from build123d import *

# Parameters (mm, degrees)
F0_W         = 190
F0_H         = 190
F0_W_2       = 11
F0_H_2       = 115.8
F0_R         = 2.1
F0_W_3       = 0.5
F0_H_3       = 0.5
F1_DEPTH     = 10
F0_W_4       = 5.2
F0_H_4       = 110
F2_DEPTH     = 5
F3_R         = 2.59999
F4_R         = 5.49999
F6_DEPTH     = 25
F8_R         = 6
F7_W         = 0.5
F7_H         = 29.5
F9_DEPTH     = 0.5
F7_W_2       = 15.563522011
F7_H_2       = 0.5
F10_DEPTH    = 0.5
F11_T2_ANGLE = 359.64
F11_T4_ANGLE = 293.7301704478
F11_T6_ANGLE = 293.7301704478


# Not quite as in the source:
# - a fillet or chamfer that OpenCascade refuses, or shapes differently, is made with other operations: its cross-section is extruded or revolved along the edge and cut away or added
# - a fillet or chamfer is up to 0.001 mm smaller than in the source, because OpenCascade refuses the exact size
# - ends of sketch curves that miss each other by under 0.0002 mm in the source are joined


with BuildPart() as f1:
    # F0 (on Top) → F1 (new body)
    with BuildSketch(Plane.XY):
        Rectangle(F0_W, F0_H)
        with BuildLine():
            ThreePointArc((50, -55), (47.0710678119, -62.0710678119), (40, -65))
            Line((40, -65), (0.25, -65))
            Line((0.25, -65), (0.25, -65.5))
            Line((0.25, -65.5), (-0.25, -65.5))
            Line((-0.25, -65.5), (-0.25, -65))
            Line((-0.25, -65), (-40, -65))
            ThreePointArc((-40, -65), (-47.0710678119, -62.0710678119), (-50, -55))
            Line((-50, -55), (-50, 55))
            ThreePointArc((-50, 55), (-47.0710678119, 62.0710678119), (-40, 65))
            Line((-40, 65), (-21, 65))
            ThreePointArc((-21, 65), (-13.9289321881, 62.0710678119), (-11, 55))
            Line((-11, 55), (-11, -9))
            ThreePointArc((-11, -9), (-7.8660663613, -16.6892782496), (-0.25, -19.997158724))
            Line((-0.25, -19.997158724), (-0.25, -19.5))
            Line((-0.25, -19.5), (0.25, -19.5))
            Line((0.25, -19.5), (0.25, -19.997158724))
            ThreePointArc((0.25, -19.997158724), (7.8660663613, -16.6892782496), (11, -9))
            Line((11, -9), (11, 55))
            ThreePointArc((11, 55), (13.9289321881, 62.0710678119), (21, 65))
            Line((21, 65), (40, 65))
            ThreePointArc((40, 65), (47.0710678119, 62.0710678119), (50, 55))
            Line((50, 55), (50, -55))
        make_face(mode=Mode.SUBTRACT)
        with Locations((-73.936477989, 0)):
            Rectangle(F0_W_2, F0_H_2, mode=Mode.SUBTRACT)
        Circle(F0_R, mode=Mode.SUBTRACT)
        with Locations((73.936477989, 0)):
            Rectangle(F0_W_2, F0_H_2, mode=Mode.SUBTRACT)
        with BuildLine():
            ThreePointArc((0, -20), (0.1250080726, -19.9992896581), (0.25, -19.997158724))
            Line((0.25, -19.997158724), (0.25, -19.5))
            Line((0.25, -19.5), (-0.25, -19.5))
            Line((-0.25, -19.5), (-0.25, -19.997158724))
            ThreePointArc((-0.25, -19.997158724), (-0.1250080726, -19.9992896581), (0, -20))
        make_face()
        with Locations((0, -65.25)):
            Rectangle(F0_W_3, F0_H_3)
    extrude(amount=F1_DEPTH)

    # F0 (on Top) → F2 (join)
    with BuildSketch(Plane.XY):
        with Locations((-73.936477989, 0)):
            Rectangle(F0_W_2, F0_H_2)
        with Locations((-73.936477989, 0)):
            Rectangle(F0_W_4, F0_H_4, mode=Mode.SUBTRACT)
        with Locations((73.936477989, 0)):
            Rectangle(F0_W_2, F0_H_2)
        with Locations((73.936477989, 0)):
            Rectangle(F0_W_4, F0_H_4, mode=Mode.SUBTRACT)
    extrude(amount=F2_DEPTH)

    # F3 (radius 2.6 in the source; OpenCascade refuses exactly that, so slightly less here)
    f3_edges = [f1.edges().sort_by_distance(p)[0] for p in [
        (-76.536478, 55, 2.5),
        (-71.336478, 55, 2.5),
        (-76.536478, -55, 2.5),
        (-71.336478, -55, 2.5),
        (76.536478, -55, 2.5),
        (71.336478, -55, 2.5),
        (71.336478, 55, 2.5),
        (76.536478, 55, 2.5),
    ]]
    fillet(f3_edges, radius=F3_R)

    # F4 (radius 5.5 in the source; OpenCascade refuses exactly that, so slightly less here)
    f4_edges = [f1.edges().sort_by_distance(p)[0] for p in [
        (-79.436478, 57.9, 7.5),
        (-68.436478, 57.9, 7.5),
        (79.436478, 57.9, 7.5),
        (68.436478, 57.9, 7.5),
        (68.436478, -57.9, 7.5),
        (79.436478, -57.9, 7.5),
        (-79.436478, -57.9, 7.5),
        (-68.436478, -57.9, 7.5),
    ]]
    fillet(f4_edges, radius=F4_R)

    # F5 (on face) → F6 (cut)
    with BuildSketch(Plane.XY.offset(5)):
        with BuildLine():
            Line((-73.686477989, -55.5), (-73.686477989, -54.9879537784))
            ThreePointArc((-73.686477989, -54.9879537784), (-73.8113279558, -54.9969866984), (-73.936467989, -55))
            ThreePointArc((-73.936467989, -55), (-74.0616280221, -54.9969866984), (-74.186477989, -54.9879537784))
            Line((-74.186477989, -54.9879537784), (-74.186477989, -55.5))
            Line((-74.186477989, -55.5), (-73.686477989, -55.5))
        make_face()
        with BuildLine():
            ThreePointArc((-73.936467989, 55), (-73.8113279558, 54.9969866984), (-73.686477989, 54.9879537784))
            Line((-73.686477989, 54.9879537784), (-73.686477989, 55.5))
            Line((-73.686477989, 55.5), (-74.186477989, 55.5))
            Line((-74.186477989, 55.5), (-74.186477989, 54.9879537784))
            ThreePointArc((-74.186477989, 54.9879537784), (-74.0616280221, 54.9969866984), (-73.936467989, 55))
        make_face()
    extrude(amount=-F6_DEPTH, mode=Mode.SUBTRACT)

    # F8
    f8_edges = [f1.edges().sort_by_distance(p)[0] for p in [
        (-95, -95, 5),
        (95, -95, 5),
        (95, 95, 5),
        (-95, 95, 5),
    ]]
    fillet(f8_edges, radius=F8_R)

    # F7 (on face) → F9 (cut)
    with BuildSketch(Plane.XY.offset(10)):
        with BuildLine():
            Line((-0.25, 95), (-0.25, 2.0850659462))
            ThreePointArc((-0.25, 2.0850659462), (0, 2.1), (0.25, 2.0850659462))
            Line((0.25, 2.0850659462), (0.25, 95))
            Line((0.25, 95), (-0.25, 95))
        make_face()
        with BuildLine():
            Line((-0.25, -2.0850659462), (-0.25, -19.6))
            Line((-0.25, -19.6), (0.25, -19.6))
            Line((0.25, -19.6), (0.25, -2.0850659462))
            ThreePointArc((0.25, -2.0850659462), (0, -2.1), (-0.25, -2.0850659462))
        make_face()
        with Locations((0, -80.25)):
            Rectangle(F7_W, F7_H)
        with BuildLine():
            Line((-0.25, -0.25), (-0.25, -2.0850659462))
            ThreePointArc((-0.25, -2.0850659462), (0, -2.1), (0.25, -2.0850659462))
            Line((0.25, -2.0850659462), (0.25, -0.25))
            Line((0.25, -0.25), (-0.25, -0.25))
        make_face()
        with BuildLine():
            Line((-0.25, 2.0850659462), (-0.25, 0.25))
            Line((-0.25, 0.25), (0.25, 0.25))
            Line((0.25, 0.25), (0.25, 2.0850659462))
            ThreePointArc((0.25, 2.0850659462), (0, 2.1), (-0.25, 2.0850659462))
        make_face()
    extrude(amount=-F9_DEPTH, mode=Mode.SUBTRACT)

    # F7 (on face) → F10 (cut)
    with BuildSketch(Plane.XY.offset(10)):
        with Locations((87.2182389945, 0)):
            Rectangle(F7_W_2, F7_H_2)
        with Locations((-87.2182389945, 0)):
            Rectangle(F7_W_2, F7_H_2)
    extrude(amount=-F10_DEPTH, mode=Mode.SUBTRACT)

    # F11: chamfer of 3 on 3 edges, made by hand

    # F11_s1 → F11_t2 (revolve, cut)
    with BuildSketch(Plane(origin=(0, 0, 0), x_dir=(0, 0, 1), z_dir=(0.0031415875, -0.9999950652, 0))):
        Polygon((10, -5.1), (7, -2.1), (10, -2.1), align=None)
    revolve(axis=Axis((0, 0, 10), (0, 0, 1)), revolution_arc=F11_T2_ANGLE, mode=Mode.SUBTRACT)

    # F11_s3 → F11_t4 (revolve, cut)
    with BuildSketch(Plane(origin=(0, 0, 0), x_dir=(0, 0, 1), z_dir=(0.9154508113, -0.4024298847, 0))):
        Polygon((10, -5.1), (7, -2.1), (10, -2.1), align=None)
    revolve(axis=Axis((0, 0, 10), (0, 0, 1)), revolution_arc=F11_T4_ANGLE, mode=Mode.SUBTRACT)

    # F11_s5 → F11_t6 (revolve, cut)
    with BuildSketch(Plane.XZ):
        Polygon((5.1, 10), (2.1, 7), (2.1, 10), align=None)
    revolve(axis=Axis((0, 0, 10), (0, 0, 1)), revolution_arc=F11_T6_ANGLE, mode=Mode.SUBTRACT)


solid = f1.part
Input: part model. Units: mm. Frame: model coordinates. A direction names the side the tool comes from. Round coordinates to 2 decimals unless told otherwise and drop trailing zeros. Write each loop counter-clockwise with the first axis right and the second up, starting at its lowest first coordinate (ties: lowest second). Pieces come first, ordered by that corner, then holes.
1) Contact query for flat-ended pins moving along their axis: P1, Ø5.5, axis at x = 72, y = -16, coming from the +Z side; P2, Ø3.5, axis at x = 0, y = 0, coming from the +Z side. Output: stop coordinate, or through.
2) Cut plane A-A (x = 37.5). Return the cut outline in (y, z).
3) Ray query, L1, parallel to Y at x = 0, z = 2; L2, parallel to X at y = 29.5, z = 4.75; L3, parallel to X at y = -27.5, z = 4.75. Return the intervals inside material, ascending.
4) Reachability of faces 4 (the flat face through (-1, -95, 5)), 5 (the cylindrical face through (77.783, -56.332, 7.535)), 6 (the flat face through (11, 23, 5)) from +Z, -Z, +X, -X, +Y, -Y: full face, straight path, thin tool, end or side. Return the list, or none.
5) Draft query along Y for faces 1 (the flat face through (95, -1, 5)), 2 (the cylindrical face through (-46.99, -62.15, 4.93)), 3 (the flat face through (-1, 95, 5)). Return one class per face: pulls with the +Y half, pulls with the -Y half, needs draft (parallel to the pull), parting line crosses it, or undercut.
6) Cut plane B-B (y = 36). Count the separate pieces of the cut face and the enclosed holes in it, then the cut area to 3 significant figures.
7) Cut plane C-C (x = 8.5). Return the cut outline in (y, z).
Geometry says:
1. P1: stops at z = 5
1. P2: passes through
2. outline: (-95, 0) - (-65, 0) - (-65, 10) - (-95, 10) - close; (65, 0) - (95, 0) - (95, 10) - (65, 10) - close
3. L1: y = -95 to -65, -20 to -2.1, 2.1 to 95
3. L2: x = -95 to -76.54, -71.34 to -50, -11 to 11, 50 to 71.34, 76.54 to 95
3. L3: x = -95 to -76.54, -71.34 to -50, 50 to 71.34, 76.54 to 95
4. face 4: +Z, -Z, +X, -X, -Y
4. face 5: +Z
4. face 6: +Z, -Z
5. face 1: needs draft
5. face 2: undercut
5. face 3: pulls with the +Y half
6. separate pieces: 5
6. enclosed holes: 0
6. area: 958 mm2
7. outline: (-95, 0) - (-65, 0) - (-65, 10) - (-95, 10) - close; (-15.98, 0) - (95, 0) - (95, 10) - (-15.98, 10) - close
